Check sheet for the drawn part. Datum: minimum x, y, z corner. Units: mm. Give positions to 0.01 mm unless a question says otherwise; leave off trailing zeros. Loops run counter-clockwise (first coordinate to the right, second up) from the corner with the lowest first, then second, coordinate; pieces in that order, holes last. Notation, with made-up numbers: M 54,38.5 L 60,38.5 A30 ccw 60,63.5 Z; hole C -15.75,59 d9. An arc over 180 degrees is marked long. Write each question's results on one line, items separated by ' | '. Start each with the question number.
1. Sectioned sample at A-A on y = 2.8. Record the cut outline in (x, z).
2. Material ranges on line 1 along X through (y, z) = (2.3, 6.5), recorded low to high.
3. Go/stop test with flat-tipped pins: pin 1 (3 mm diameter, centred on x = 335, y = 2.5, fed in from +Z); pin 2 (3 mm diameter, centred on y = 4, z = 36, fed in from -X); pin 3 (1.8 mm diameter, centred on y = 2.5, z = 59, fed in from +X). Record where each tip stops, or that it passes through.
4. Sectioned sample at B-B on z = 31. Record the cut outline in (x, y).
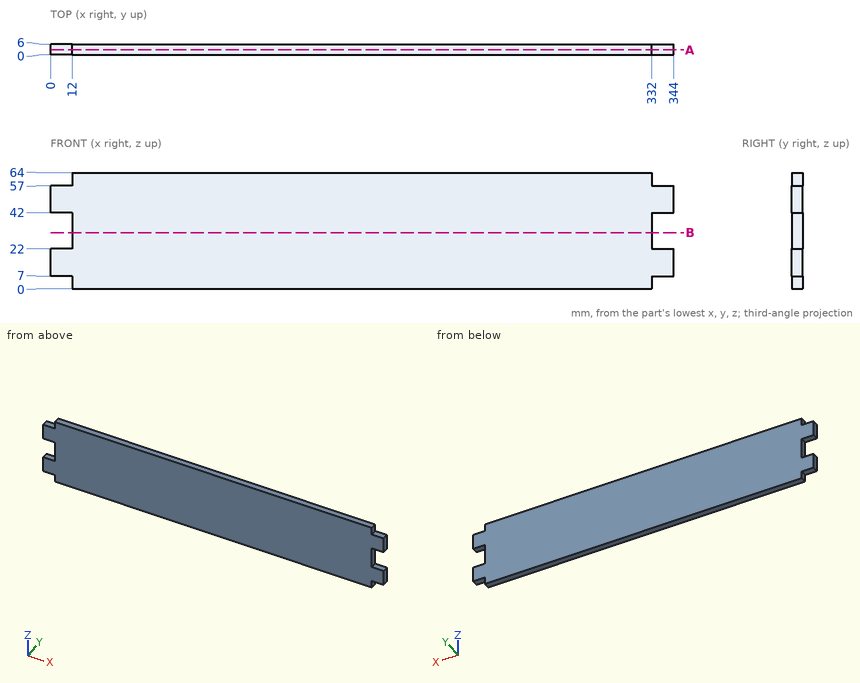
Output values:
1) outline: M 0,7 L 12,7 L 12,0 L 332,0 L 332,7 L 344,7 L 344,22 L 332,22 L 332,42 L 344,42 L 344,57 L 332,57 L 332,64 L 12,64 L 12,57 L 0,57 L 0,42 L 12,42 L 12,22 L 0,22 Z
2) line 1: 12 to 332
3) pin 1: z = 57 | pin 2: x = 12 | pin 3: x = 332
4) outline: M 12,0 L 332,0 L 332,6 L 12,6 Z
